Model file for the job. Use its own axes, mm. Face numbers are marked on the shaded views. A direction names the side the tool comes from. Give positions to 0.01 mm unless a question says otherwise; leave off trailing zeros. Loops run counter-clockwise (first coordinate to the right, second up) from the corner with the lowest first, then second, coordinate; pieces in that order, holes last. Notation, with made-up numbers: (78.5, -14) - (133.5, -14) arc R23 ccw to (133.5, 20) - close; hole circle Ø4 at (14.5, -23). An arc over 180 degrees is marked (long way). Use a Markdown table: item, result.
from build123d import *

# Parameters (mm, degrees)
SKETCH1_R               = 38.1
SKETCH1_R_2             = 9.546666028
BOSS_EXTRUDE1_DEPTH     = 38.1
SKETCH2_W               = 38.1
SKETCH2_H               = 19.05
CUT_EXTRUDE1_DEPTH      = 144.78
CUT_EXTRUDE2_DEPTH      = 22.86
CUT_EXTRUDE2_DEPTH_BACK = 20.32
SKETCH5_W               = 40.342749465
SKETCH5_H               = 23.10958947
CUT_EXTRUDE4_DEPTH      = 53.594
CUT_EXTRUDE5_DEPTH      = 10


with BuildPart() as part:
    # Sketch1 → Boss-Extrude1 (new body)
    with BuildSketch(Plane(origin=(0, 0, 0), x_dir=(1, 0, 0), z_dir=(0, 1, 0))):
        Circle(SKETCH1_R)
        Circle(SKETCH1_R_2, mode=Mode.SUBTRACT)
    extrude(amount=BOSS_EXTRUDE1_DEPTH)

    # Sketch2 → Cut-Extrude1 (cut)
    with BuildSketch(Plane.XY.offset(38.1)):
        with Locations((19.05, 9.525)):
            Rectangle(SKETCH2_W, SKETCH2_H)
    extrude(amount=-CUT_EXTRUDE1_DEPTH, mode=Mode.SUBTRACT)

    # Sketch3 → Cut-Extrude2 (cut, two sides)
    with BuildSketch(Plane.XZ.offset(-19.05)) as cut_extrude2_sk:
        with BuildLine():
            Line((0, -19.2), (-32.908509538, -19.2))
            ThreePointArc((-32.908509538, -19.2), (38.1, 0), (-32.908509538, 19.2))
            Line((-32.908509538, 19.2), (0, 19.2))
            ThreePointArc((0, 19.2), (19.2, 0), (0, -19.2))
        make_face()
    extrude(amount=CUT_EXTRUDE2_DEPTH, mode=Mode.SUBTRACT)
    extrude(cut_extrude2_sk.sketch, amount=-CUT_EXTRUDE2_DEPTH_BACK, mode=Mode.SUBTRACT)

    # Sketch5 → Cut-Extrude4 (cut)
    with BuildSketch(Plane.XY.offset(19.2)):
        with Locations((-20.171374733, 7.495205265)):
            Rectangle(SKETCH5_W, SKETCH5_H)
    extrude(amount=-CUT_EXTRUDE4_DEPTH, mode=Mode.SUBTRACT)

    # Sketch6 → Cut-Extrude5 (cut)
    with BuildSketch(Plane(origin=(0, 38.1, 0), x_dir=(1, 0, 0), z_dir=(0, 1, 0))):
        with BuildLine():
            Line((-19.2, 19.2), (-19.2, -19.2))
            Line((-19.2, -19.2), (-32.908509538, -19.2))
            ThreePointArc((-32.908509538, -19.2), (-38.1, 0), (-32.908509538, 19.2))
            Line((-32.908509538, 19.2), (-19.2, 19.2))
        make_face()
    extrude(amount=-CUT_EXTRUDE5_DEPTH, mode=Mode.SUBTRACT)


solid = part.part
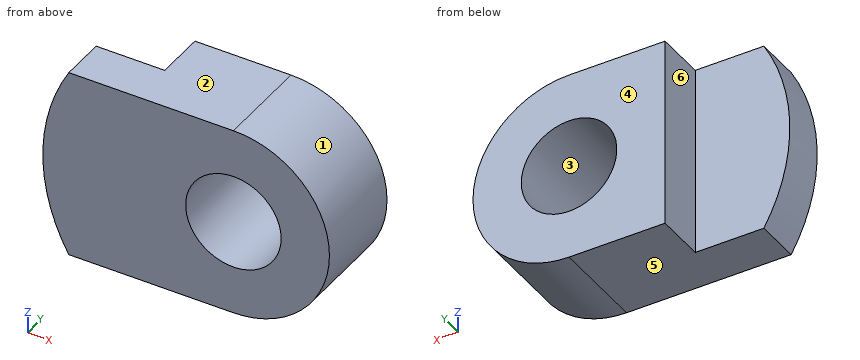
(1) Drill centre lines: probe 1 along X at (y, z) = (29, 0); probe 2 along Y at (x, z) = (-31, -7); probe 3 along Z at (x, y) = (5.5, 27). Where is each one in solid material? Low to high. Write a range as [from, to].
Computed:
| item | result |
|---|---|
| probe 1 | [-19.2, -9.55], [9.55, 19.2] |
| probe 2 | [19.05, 28.1] |
| probe 3 | [-18.4, -7.8], [7.8, 18.4] |
(2) 3-axis set-ups, long thin cutter, end or side, ignore diameter. For the marked faces 5 and 6: which of +Z, -Z, +X, -X, +Y, -Y reach the whole face in a straight line?
Computed:
| item | result |
|---|---|
| face 5 | -Z, +X, -X, +Y, -Y |
| face 6 | +Z, -Z, -X, +Y |
(3) Slice it at C-C, the plane x = -7. Write the cut outline in (y, z), plus the area to 3 significant figures.
Computed:
| item | result |
|---|---|
| outline | (19.05, -19.2) - (38.1, -19.2) - (38.1, -6.49) - (19.05, -6.49) - close; (19.05, 6.49) - (38.1, 6.49) - (38.1, 19.2) - (19.05, 19.2) - close |
| area | 484 mm² |
(4) Slice it at D-D, the plane z = -4. Write the cut outline in (x, y), plus the area to 3 significant figures.
Computed:
| item | result |
|---|---|
| outline | (-37.89, 19.05) - (-8.67, 19.05) - (-8.67, 38.1) - (-19.2, 38.1) - (-19.2, 28.1) - (-37.89, 28.1) - close; (8.67, 19.05) - (18.78, 19.05) - (18.78, 38.1) - (8.67, 38.1) - close |
| area | 562 mm² |
(5) Slice it at A-A, the plane z = 0. Write the cut outline in (x, y).
Computed:
| item | result |
|---|---|
| outline | (-38.1, 19.05) - (-9.55, 19.05) - (-9.55, 38.1) - (-19.2, 38.1) - (-19.2, 28.1) - (-38.1, 28.1) - close; (9.55, 19.05) - (19.2, 19.05) - (19.2, 38.1) - (9.55, 38.1) - close |
(6) Pin check, flat tips, straight feed: P1, Ø10, axis at y = 35, z = -4.5, coming from the -X side; P2, Ø1, axis at y = 21.5, z = -11, coming from the +X side; P3, Ø3, axis at y = 24, z = 3.5, coming from the +X side. Stop position of each tip, or through.
Computed:
| item | result |
|---|---|
| P1 | x = -19.2 |
| P2 | x = 16.07 |
| P3 | x = 19.1 |
(7) Slice it at B-B, the plane y = 32.5. Write the cut outline in (x, z), plus the area to 3 significant figures.
Computed:
| item | result |
|---|---|
| outline | (-19.2, -19.2) - (0, -19.2) arc R19.2 ccw to (0, 19.2) - (-19.2, 19.2) - close; hole circle Ø19.09 at (0, 0) |
| area | 1,030 mm² |
(8) Mould opens along Z. For the marked faces 1, 2, 3 and 4 say: pulls with the +Z half, pulls with the -Z half, needs draft (parallel to the pull), parting line crosses it, or undercut.
Computed:
| item | result |
|---|---|
| face 1 | parting line crosses it |
| face 2 | pulls with the +Z half |
| face 3 | undercut |
| face 4 | needs draft |
